```python
from build123d import *

# Parameters (mm, degrees)
SKETCH1_R                = 115
SKETCH1_R_2              = 105.05
BOSS_EXTRUDE1_DEPTH      = 40
BOSS_EXTRUDE2_DEPTH      = 40
FILLET2_R                = 1
CIRPATTERN2_COUNT        = 8
FILLET2_OF_CIRPATTERN2_R = 1
CUT_EXTRUDE2_DEPTH       = 41


with BuildPart() as part:
    # Sketch1 → Boss-Extrude1 (new body)
    with BuildSketch(Plane(origin=(0, 0, 0), x_dir=(1, 0, 0), z_dir=(0, 1, 0))):
        Circle(SKETCH1_R)
        Circle(SKETCH1_R_2, mode=Mode.SUBTRACT)
    extrude(amount=BOSS_EXTRUDE1_DEPTH)

    # Sketch2 → Boss-Extrude2 (add, through all)
    with BuildSketch(Plane(origin=(0, 40, 0), x_dir=(1, 0, 0), z_dir=(0, 1, 0))):
        with BuildLine():
            ThreePointArc((2.891374007, 105.010201678), (0, 105.05), (-2.891374007, 105.010201678))
            Line((-2.891374007, 105.010201678), (-5.889932008, 97.372024735))
            ThreePointArc((-5.889932008, 97.372024735), (0, 97.55), (5.889932008, 97.372024735))
            Line((5.889932008, 97.372024735), (2.891374007, 105.010201678))
        make_face()
    boss_extrude2 = extrude(amount=-BOSS_EXTRUDE2_DEPTH)

    # Fillet2
    fillet2_edges = [part.edges().sort_by_distance(p)[0] for p in [
        (5.889932008, 20, -97.372024735),
        (-5.889932008, 20, -97.372024735),
        (-2.891374007, 20, -105.010201678),
        (2.891374007, 20, -105.010201678),
    ]]
    fillet(fillet2_edges, radius=FILLET2_R)

    # CirPattern2: Boss-Extrude2 ×8 about axis
    cirpattern2_axis = Axis((0, 0, 0), (0, 1, 0))
    for i in range(1, CIRPATTERN2_COUNT):
        add(boss_extrude2.rotate(cirpattern2_axis, i * 360 / CIRPATTERN2_COUNT))

    # Fillet2 of CirPattern2
    fillet2_of_cirpattern2_edges = [part.edges().sort_by_distance(p)[0] for p in [
        (-64.687608124, 20, -73.017229852),
        (-73.017229852, 20, -64.687608124),
        (-76.297935867, 20, -72.208915532),
        (-72.208915532, 20, -76.297935867),
        (-97.372024735, 20, -5.889932008),
        (-97.372024735, 20, 5.889932008),
        (-105.010201678, 20, 2.891374007),
        (-105.010201678, 20, -2.891374007),
        (-73.017229852, 20, 64.687608124),
        (-64.687608124, 20, 73.017229852),
        (-72.208915532, 20, 76.297935867),
        (-76.297935867, 20, 72.208915532),
        (-5.889932008, 20, 97.372024735),
        (5.889932008, 20, 97.372024735),
        (2.891374007, 20, 105.010201678),
        (-2.891374007, 20, 105.010201678),
        (64.687608124, 20, 73.017229852),
        (73.017229852, 20, 64.687608124),
        (76.297935867, 20, 72.208915532),
        (72.208915532, 20, 76.297935867),
        (97.372024735, 20, 5.889932008),
        (97.372024735, 20, -5.889932008),
        (105.010201678, 20, -2.891374007),
        (105.010201678, 20, 2.891374007),
        (73.017229852, 20, -64.687608124),
        (64.687608124, 20, -73.017229852),
        (72.208915532, 20, -76.297935867),
        (76.297935867, 20, -72.208915532),
    ]]
    fillet(fillet2_of_cirpattern2_edges, radius=FILLET2_OF_CIRPATTERN2_R)

    # Sketch3 → Cut-Extrude2 (cut, through all)
    with BuildSketch(Plane(origin=(0, 40, 0), x_dir=(1, 0, 0), z_dir=(0, 1, 0))):
        with BuildLine():
            Line((-0.15, 117.349449893), (-0.15, -117.349449893))
            ThreePointArc((-0.15, -117.349449893), (82.828591788, -82.978591788), (117.199449893, 0))
            ThreePointArc((117.199449893, 0), (82.828591788, 82.978591788), (-0.15, 117.349449893))
        make_face()
    extrude(amount=-CUT_EXTRUDE2_DEPTH, mode=Mode.SUBTRACT)


solid = part.part
```
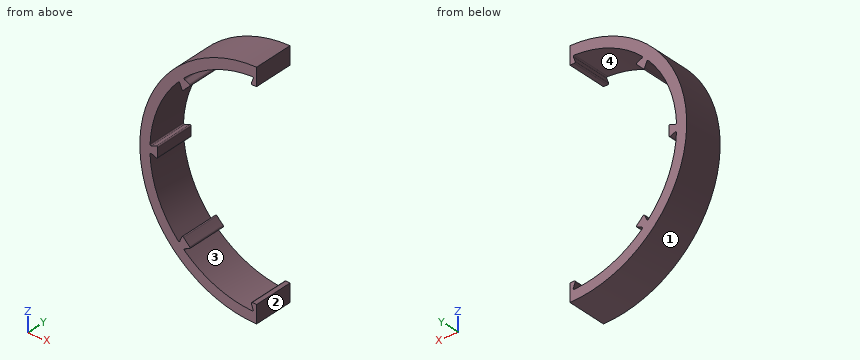
Check sheet for the modelled part. Datum: model origin and axes. Units: mm. Face numbers are marked on the shaded views. Round coordinates to 2 decimals unless told otherwise and drop trailing zeros. Write each loop counter-clockwise with the first axis right and the second up, starting at its lowest first coordinate (ties: lowest second). Pieces come first, ordered by that corner, then holes. Notation, with made-up numbers: M 48.25,-15.75 L 85.25,-15.75 A8 cw 85.25,-1.75 Z; hole C -17,8 d7. An arc over 180 degrees is marked long. Write item = value, one per line. Start each with the question number.
1. Scan lines: line 1 (Z direction, x = -57, y = 3); line 2 (X direction, y = 18, z = -67.5); line 3 (Z direction, x = -40, y = 23). Record each from-to range of solid material in increasing order. Write a range as [from, to].
2. Section check C-C, the plane x = -28.5. Record the cut outline in (y, z).
3. Gauge pin test, flat ends, axial feed: pin 1 (2 mm diameter, centred on x = -21.5, y = 18, fed in from +Z); pin 2 (12 mm diameter, centred on x = -17.5, y = 12, fed in from +Z); pin 3 (1 mm diameter, centred on y = 8.5, z = -27.5, fed in from -X). Record the tip position at first contact, or that the pin passes through.
4. Release check for a two-part mould opening along X. For the marked faces 1, 2, 3 and 4 record: pulls with the +X half, pulls with the -X half, needs draft (parallel to the pull), parting line crosses it, or undercut.
5. Section check B-B, the plane z = 0. Record the cut outline in (x, y).
6. Section check A-A, the plane x = -61. Record the cut outline in (y, z).
Results found:
q1.line_1 = [-99.88, -88.24], [88.24, 99.88]
q1.line_2 = [-93.11, -80.49], [-74.24, -70.43]
q1.line_3 = [-107.82, -97.14], [97.14, 107.82]
q2.outline = M 0,-111.41 L 40,-111.41 L 40,-101.11 L 0,-101.11 Z; M 0,101.11 L 40,101.11 L 40,111.41 L 0,111.41 Z
q3.pin_1 = 113.16
q3.pin_2 = 114.42
q3.pin_3 = -111.79
q4.face_1 = pulls with the -X half
q4.face_2 = pulls with the +X half
q4.face_3 = undercut
q4.face_4 = undercut
q5.outline = M -115,0 L -97.55,0 L -97.55,40 L -115,40 Z
q6.outline = M 0,-97.49 L 40,-97.49 L 40,-85.52 L 0,-85.52 Z; M 0,85.52 L 40,85.52 L 40,97.49 L 0,97.49 Z
